CAD build for the part. Positions are in the model's coordinates, mm. A direction names the side the tool comes from. Round coordinates to 2 decimals unless told otherwise and drop trailing zeros. Order: outer loops, then holes, each group sorted by start corner. A loop starts at its lowest first (then second) coordinate and runs counter-clockwise, first axis right, second up. Notation, with made-up numbers: (-34.5, 45) -> (-15.5, 45) arc R37 ccw to (-15.5, 83) -> close; hole circle Ø10 at (-32, 0). An arc over 180 degrees is marked (long way). Return JSON: item names as keys, results as strings. Group by question number.
Q1. Cut at D-D (x = 16). Write the cut outline in (y, z), then the cut area to 3 significant figures.
Q2. Mould opens along X. For faces 1 (the flat face through (6, -10, 4)), 2 (the cylindrical face through (-0.779, -26.445, 1.972)), 3 (the flat face through (6.5, -18, 2)) say: +X half, -X half, draft (parallel to the pull), parting line (faces both ways), or undercut.
Q3. Cut at A-A (x = 0). Write the cut outline in (y, z).
Q4. Which spindle directions (+Z, -Z, +X, -X, +Y, -Y) get a long thin tool onto all of the face, cutting with end or side? Do faces 4 (the flat face through (22, -17, 2)), 5 (the flat face through (22, -9.2, 2)), 6 (the flat face through (11.5, -19, 2)), 7 (the cylindrical face through (5.3, -4.22, 1.97)). Say none if no direction does.
Q5. Cut at C-C (z = 0.6). Write the cut outline in (x, y) (3 decimals).
Q6. Probe line 1 along Y through (x, z) = (0, 0.9); line 2 along Y through (x, z) = (13, 3.6); line 3 along Y through (x, z) = (8.5, 3.5). List the from-to ranges inside material, lowest first.
Q7. Flat gauge pins, fed straight in: pin 1 (8 mm diameter, centred on x = 16, y = 1, fed in from -Z); pin 2 (2 mm diameter, centred on y = -19.5, z = 1.5, fed in from +X); pin 3 (1.5 mm diameter, centred on x = 14.5, z = 2.5, fed in from -Y); pin 4 (2 mm diameter, centred on x = 21.5, z = 2.5, fed in from -Y). Where does each tip first touch, or does it go through?
Q8. Cut at B-B (y = -0.5). Write the cut outline in (x, z), then the cut area to 3 significant figures.
from build123d import *

# Parameters (mm, degrees)
SKETCH1_R           = 1.5
BOSS_EXTRUDE1_DEPTH = 4
SKETCH2_W           = 5
SKETCH2_H           = 5
CUT_EXTRUDE1_DEPTH  = 4


with BuildPart() as part:
    # Sketch1 → Boss-Extrude1 (new body)
    with BuildSketch(Plane.XY):
        with BuildLine():
            Line((11.5, -1.2), (11.5, -9.2))
            ThreePointArc((11.5, -9.2), (6.499964862, -6.763292795), (5.338318884, -1.323764138))
            ThreePointArc((5.338318884, -1.323764138), (0.016750191, 5.499974494), (-5.34628284, -1.291224148))
            ThreePointArc((-5.34628284, -1.291224148), (-4.25, -10.5), (-5.34628284, -19.708775852))
            ThreePointArc((-5.34628284, -19.708775852), (-0.650170894, -26.461435508), (5.5, -21))
            ThreePointArc((5.5, -21), (6.671572875, -18.171572875), (9.5, -17))
            Line((9.5, -17), (11.5, -17))
            Line((11.5, -17), (11.5, -21))
            Line((11.5, -21), (19.5, -21))
            Line((19.5, -21), (19.5, -17))
            Line((19.5, -17), (24.5, -17))
            Line((24.5, -17), (24.5, -9.2))
            Line((24.5, -9.2), (19.5, -9.2))
            Line((19.5, -9.2), (19.5, -1.2))
            Line((19.5, -1.2), (11.5, -1.2))
        make_face()
        Circle(SKETCH1_R, mode=Mode.SUBTRACT)
        with Locations((0, -21)):
            Circle(SKETCH1_R, mode=Mode.SUBTRACT)
    extrude(amount=BOSS_EXTRUDE1_DEPTH)

    # Sketch2 → Cut-Extrude1 (cut)
    with BuildSketch(Plane.XY.offset(4)):
        with Locations((9, -6.7)):
            Rectangle(SKETCH2_W, SKETCH2_H)
        with Locations((9, -19.5)):
            Rectangle(SKETCH2_W, SKETCH2_H)
    extrude(amount=-CUT_EXTRUDE1_DEPTH, mode=Mode.SUBTRACT)


solid = part.part
Solution:
{
 "1": {"outline": "(-21, 0) -> (-1.2, 0) -> (-1.2, 4) -> (-21, 4) -> close", "area": "79.2 mm²"},
 "2": {"face 1": "draft", "face 2": "parting line", "face 3": "undercut"},
 "3": {"outline": "(-26.5, 0) -> (-22.5, 0) -> (-22.5, 4) -> (-26.5, 4) -> close; (-19.5, 0) -> (-1.5, 0) -> (-1.5, 4) -> (-19.5, 4) -> close; (1.5, 0) -> (5.5, 0) -> (5.5, 4) -> (1.5, 4) -> close"},
 "4": {"face 4": "+Z, -Z, +X, -Y", "face 5": "+Z, -Z, +X, +Y", "face 6": "+Z, -Z, -Y", "face 7": "+Z, -Z"},
 "5": {"outline": "(-5.346, -19.709) arc R5.5 ccw (long way) to (5.5, -21) arc R4 cw to (6.5, -18.354) -> (6.5, -17) -> (11.5, -17) -> (11.5, -21) -> (19.5, -21) -> (19.5, -17) -> (24.5, -17) -> (24.5, -9.2) -> (19.5, -9.2) -> (19.5, -1.2) -> (11.5, -1.2) -> (11.5, -9.2) -> (6.5, -9.2) -> (6.5, -6.763) arc R6.348 cw to (5.338, -1.324) arc R5.5 ccw (long way) to (-5.346, -1.291) arc R39.225 cw to start; hole circle Ø3 at (0, -21); hole circle Ø3 at (0, 0)"},
 "6": {"line 1": "y = -26.5 to -22.5, -19.5 to -1.5, 1.5 to 5.5", "line 2": "y = -21 to -1.2", "line 3": "y = -17 to -9.2"},
 "7": {"pin 1": "stops at z = 0", "pin 2": "stops at x = 19.5", "pin 3": "stops at y = -21", "pin 4": "stops at y = -17"},
 "8": {"outline": "(-5.48, 0) -> (-1.41, 0) -> (-1.41, 4) -> (-5.48, 4) -> close; (1.41, 0) -> (5.48, 0) -> (5.48, 4) -> (1.41, 4) -> close", "area": "32.5 mm²"}
}
